Geometry check sheet. Reference: the model listing, model coordinates, mm. Face numbers are marked on the shaded views. A direction names the side the tool comes from. Give positions to 0.01 mm unless a question says otherwise; leave off trailing zeros. Write each loop counter-clockwise with the first axis right and the second up, starting at its lowest first coordinate (ties: lowest second). Pieces come first, ordered by that corner, then holes. Notation, with made-up numbers: (30.5, 63) -> (45.5, 63) arc R21 cw to (45.5, 94) -> close; hole circle Ø7 at (-26.5, 44.25). An arc over 180 degrees is marked (long way). Use a Markdown table: item, result. Add a question column.
Autodesk Inventor part; units mm, degrees
ref_plane "YZ Plane" through (0, 0, 0) normal (1, 0, 0) x (0, 1, 0)
ref_plane "XZ Plane" through (0, 0, 0) normal (0, 1, 0) x (-1, 0, 0)
ref_plane "XY Plane" through (0, 0, 0) normal (0, 0, 1) x (1, 0, 0)
ref_plane "Work Plane1" through (182.8917, 65.9403, 21.7484) normal (0, 1, 0) x (0, 0, -1)
sketch "Sketch1" plane through (182.8917, 65.9403, 21.7484) normal (0, 1, 0) x (0, 0, -1)
  line L0 (-78.6913, -1.8576) -> (-78.6913, -56.8576)
  line L1 (-78.6913, -56.8576) -> (-75.6913, -56.8576)
  line L2 (-75.6913, -56.8576) -> (-75.6913, -31.8576)
  line L3 (-75.6913, -31.8576) -> (-28.6913, -31.8576)
  line L4 (-28.6913, -31.8576) -> (-28.6913, -28.8576)
  line L5 (-28.6913, -31.8576) -> (-28.6913, -51.8576)
  line L6 (-28.6913, -51.8576) -> (-25.6913, -51.8576)
  line L7 (-25.6913, -51.8576) -> (-25.6913, -28.8576)
  line L8 (-25.6913, -28.8576) -> (-75.6913, -28.8576)
  line L9 (-75.6913, -28.8576) -> (-75.6913, -1.8576)
  line L10 (-75.6913, -1.8576) -> (-78.6913, -1.8576)
  point P0 (21.7484, 182.8917)
  dimension "d0" = 55
  dimension "d1" = 3
  dimension "d2" = 25
  dimension "d3" = 47
  dimension "d4" = 3
  dimension "d5" = 3
  dimension "d6" = 23
extrude "Extrusion1" add sketch "Sketch1" along normal blind 6.8
properties part number "battery_holder_3DPrint"
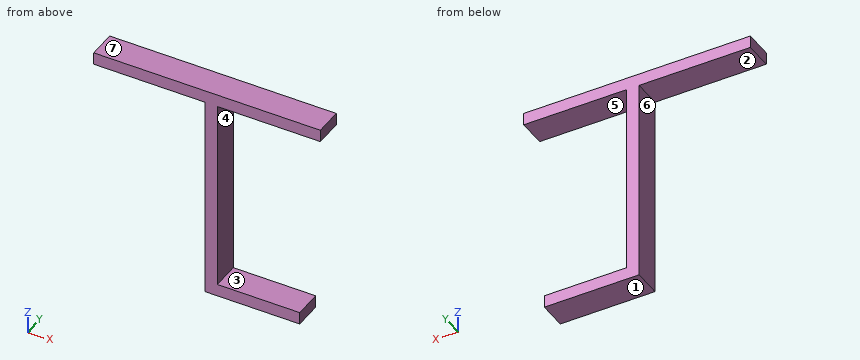
1) Sectioned sample at D-D, the plane x = 204. Enter the section's corners in (y, z), and give its area (3 significant figures).
2) Draft check along Z on the marked faces 4, 5, 6 and 7. Enter one of: +Z half, -Z half, draft (parallel to the pull), parting line (faces both ways), or undercut.
3) Gauge pin test, flat end, axial feed: P1, Ø2.5, axis at y = 71, z = 49, coming from the +X side. Record the tip position at first contact, or that the pin passes through.
4) Material ranges on probe 1 along Z at (x, y) = (217, 68.25); probe 2 along Z at (x, y) = (187.5, 66.5); probe 3 along X at (y, z) = (69.5, 89), recorded low to high. Write a range as [from, to].
5) Tool access check on the marked faces 1, 2 and 3. Record the directions out of +Z, -Z, +X, -X, +Y, -Y that give a thin tool (end or side, any length) a straight path to the whole face; none if there is none.
6) Sectioned sample at A-A, the plane x = 233. Enter the section's corners in (y, z), and give its area (3 significant figures).
7) Sectioned sample at C-C, the plane z = 96.5. Enter the section's corners in (x, y), and give its area (3 significant figures).
8) Sectioned sample at B-B, the plane y = 69.5. Enter the section's corners in (x, z), and give its area (3 significant figures).
Check values:
| question | item | result |
|---|---|---|
| 1 | outline | (65.94, 97.44) -> (72.74, 97.44) -> (72.74, 100.44) -> (65.94, 100.44) -> close |
| 1 | area | 20.4 mm² |
| 2 | face 4 | undercut |
| 2 | face 5 | undercut |
| 2 | face 6 | draft |
| 2 | face 7 | +Z half |
| 3 | P1 | x = 234.75 |
| 4 | probe 1 | [47.44, 50.44], [97.44, 100.44] |
| 4 | probe 2 | [97.44, 100.44] |
| 4 | probe 3 | [211.75, 214.75] |
| 5 | face 1 | -Z, +X, -X, +Y, -Y |
| 5 | face 2 | -Z, -X, +Y, -Y |
| 5 | face 3 | +X, +Y, -Y |
| 6 | outline | (65.94, 47.44) -> (72.74, 47.44) -> (72.74, 50.44) -> (65.94, 50.44) -> close; (65.94, 97.44) -> (72.74, 97.44) -> (72.74, 100.44) -> (65.94, 100.44) -> close |
| 6 | area | 40.8 mm² |
| 7 | outline | (211.75, 65.94) -> (214.75, 65.94) -> (214.75, 72.74) -> (211.75, 72.74) -> close |
| 7 | area | 20.4 mm² |
| 8 | outline | (184.75, 97.44) -> (211.75, 97.44) -> (211.75, 47.44) -> (234.75, 47.44) -> (234.75, 50.44) -> (214.75, 50.44) -> (214.75, 97.44) -> (239.75, 97.44) -> (239.75, 100.44) -> (184.75, 100.44) -> close |
| 8 | area | 375 mm² |
